```python
from build123d import *

# Parameters (mm, degrees)
SKETCH1_R           = 10
SHAFT_D20X100_DEPTH = 100
SKETCH3_W           = 6
SKETCH3_H           = 3
KEYWAY_6X25_DEPTH   = 25
SKETCH4_W           = 6
SKETCH4_H           = 3
KEYWAT2_6X25_DEPTH  = 25


with BuildPart() as part:
    # Sketch1 → Shaft_D20x100 (new body)
    with BuildSketch(Plane.XY):
        with Locations(Location((0, 0, 0), (0, 0, 180))):
            Circle(SKETCH1_R)
    extrude(amount=SHAFT_D20X100_DEPTH)

    # Sketch3 → Keyway_6x25 (cut)
    with BuildSketch(Plane(origin=(0, 0, 0), x_dir=(-1, 0, 0), z_dir=(0, 0, -1))):
        with Locations((0.706795811, 8.5)):
            Rectangle(SKETCH3_W, SKETCH3_H)
    extrude(amount=-KEYWAY_6X25_DEPTH, mode=Mode.SUBTRACT)

    # Sketch4 → keywat2_6x25 (cut)
    with BuildSketch(Plane.XY.offset(100)):
        with Locations((0.063890127, 8.5)):
            Rectangle(SKETCH4_W, SKETCH4_H)
    extrude(amount=-KEYWAT2_6X25_DEPTH, mode=Mode.SUBTRACT)


solid = part.part
```
Read the model definition and answer for the solid it produces. Units are mm, in the model's axes. A direction names the side the tool comes from. Coordinates: 2 decimals unless noted, no trailing zeros. Write each loop counter-clockwise with the first axis right and the second up, starting at its lowest first coordinate (ties: lowest second). Pieces come first, ordered by that corner, then holes. Notation, with made-up numbers: (-23, 13.25) - (22, 13.25) arc R8 cw to (22, 24.25) - close; hole circle Ø11 at (47.25, 52). An arc over 180 degrees is marked (long way). Answer as a JSON object with one key per item and string values. Group by question number.
1. A cutting plane is placed at C-C (y = -8). Determine the outline of the cut face in (x, z).
2. The mould has two halves that part along X. Classify faces 1 (the flat face through (0, 7, 88)), 2 (the cylindrical face through (1.302, -9.915, 49.3)), 3 (the flat face through (0, 0, 0)): +X half, -X half, draft (parallel to the pull), parting line (faces both ways), or undercut.
3. A cutting plane is placed at D-D (z = 21). Determine the outline of the cut face in (x, y).
4. A cutting plane is placed at A-A (x = 0). Determine the outline of the cut face in (y, z), plus the area to 3 significant figures.
5. Consider L1, parallel to X at y = 7.75, z = 84; L2, parallel to Y at x = -0.5, z = 65.5; L3, parallel to Y at x = 4.25, z = 39. Determine where each line is inside the solid, lowest interval first. Write a range as [from, to].
6. Which of the six approach directions +Z, -Z, +X, -X, +Y, -Y give full straight-line access (tool end or side, diameter ignored) to faces 4 (the flat face through (0, 9, 75)), 5 (the flat face through (0, 0, 100)), 6 (the flat face through (2.293, 8, 12))?
7. A cutting plane is placed at B-B (z = 40). Determine the outline of the cut face in (x, y).
8. Each of these flat-tipped pins is pushed along its axis until it touches: P1, Ø1, axis at y = 2, z = 29, coming from the -X side; P2, Ø0.9, axis at x = -0.5, y = 8.5, coming from the -Z side; P3, Ø1.4, axis at y = 8.5, z = 12.5, coming from the -X side. Where does it stop, or does it pass through?
Worked out:
{
 "1": {"outline": "(-6, 0) - (6, 0) - (6, 100) - (-6, 100) - close"},
 "2": {"face 1": "undercut", "face 2": "parting line", "face 3": "draft"},
 "3": {"outline": "(-3.71, 7) - (-3.71, 9.29) arc R10 ccw (long way) to (2.29, 9.73) - (2.29, 7) - close"},
 "4": {"outline": "(-10, 0) - (7, 0) - (7, 25) - (10, 25) - (10, 75) - (7, 75) - (7, 100) - (-10, 100) - close", "area": "1,850 mm²"},
 "5": {"L1": "x = [-6.32, -2.94], [3.06, 6.32]", "L2": "y = [-9.99, 9.99]", "L3": "y = [-9.05, 9.05]"},
 "6": {"face 4": "+Z, +Y", "face 5": "+Z, +X, -X, +Y, -Y", "face 6": "-Z, +Y"},
 "7": {"outline": "circle Ø20 at (0, 0)"},
 "8": {"P1": "stops at x = -9.89", "P2": "stops at z = 25", "P3": "stops at x = -6.26"}
}
